Autodesk Inventor part; units mm, degrees
ref_plane "YZ Plane" through (0, 0, 0) normal (1, 0, 0) x (0, 1, 0)
ref_plane "XZ Plane" through (0, 0, 0) normal (0, 1, 0) x (-1, 0, 0)
ref_plane "XY Plane" through (0, 0, 0) normal (0, 0, 1) x (1, 0, 0)
sketch "Sketch1" plane through (0, 0, 0) normal (0, 0, 1) x (1, 0, 0)
  line L0 (-14, -0.25) -> (0, -0.25)
  line L1 (0, -0.25) -> (0, 0)
  line L2 (0, 0) -> (0, 10)
  line L3 (0, 10) -> (0, 10.25)
  line L4 (0, 10.25) -> (-14, 10.25)
  line L5 (-14, 10.25) -> (-14, -0.25)
  circle A0 centre (-7, 5) radius 1.5
  line L6 (0, 0) -> (-14, 0)
  line L7 (-14, 0) -> (-14, 10)
  line L8 (-14, 10) -> (0, 10)
  line L9 (0, 10) -> (0, 0)
  dimension "d0" = 0.25
  dimension "d1" = 0.25
extrude "Extrusion1" add sketch "Sketch1" along normal blind 1.5 contours L5 L8 L2 L6
properties part number "arm_plate"
Input: part model. Units: mm. Frame: model coordinates. Coordinates: 2 decimals unless noted, no trailing zeros. Loops run counter-clockwise (first coordinate to the right, second up) from the corner with the lowest first, then second, coordinate; pieces in that order, holes last.
Q1. Cut plane A-A (x = -7). Output: boundary loops of the cut face in (y, z).
Q2. Cut plane C-C (z = 0.85). Output: boundary loops of the cut face in (x, y).
Q3. Cut plane B-B (y = 5). Output: boundary loops of the cut face in (x, z), then the cut area to 3 significant figures.
Q4. Contact query for a flat-ended pin moving along its axis: pin 1 (2 mm diameter, centred on x = -7.5, y = 5.5, fed in from +Z). Output: stop coordinate, or through.
Q5. Draft query along Y for faces 1 (the face through (-7, 0, 1)), 2 (the face through (-8.5, 4.93, 0.74)), 3 (the face through (-9, 5, 1.5)). Return one class per face: +Y half, -Y half, draft (parallel to the pull), parting line (faces both ways), or undercut.
Q6. Material intervals for line 1 (Y direction, x = -7, z = 0.6); line 2 (Y direction, x = -8.25, z = 1.4); line 3 (X direction, y = 5.75, z = 1.15), sorted ascending.
Working result:
1. outline: (0, 0) - (3.5, 0) - (3.5, 1.5) - (0, 1.5) - close; (6.5, 0) - (10, 0) - (10, 1.5) - (6.5, 1.5) - close
2. outline: (-14, 0) - (0, 0) - (0, 10) - (-14, 10) - close; hole circle Ø3 at (-7, 5)
3. outline: (-14, 0) - (-8.5, 0) - (-8.5, 1.5) - (-14, 1.5) - close; (-5.5, 0) - (0, 0) - (0, 1.5) - (-5.5, 1.5) - close
3. area: 16.5 mm2
4. pin 1: stops at z = 1.5
5. face 1: -Y half
5. face 2: undercut
5. face 3: draft
6. line 1: y = 0 to 3.5, 6.5 to 10
6. line 2: y = 0 to 4.17, 5.83 to 10
6. line 3: x = -14 to -8.3, -5.7 to 0
